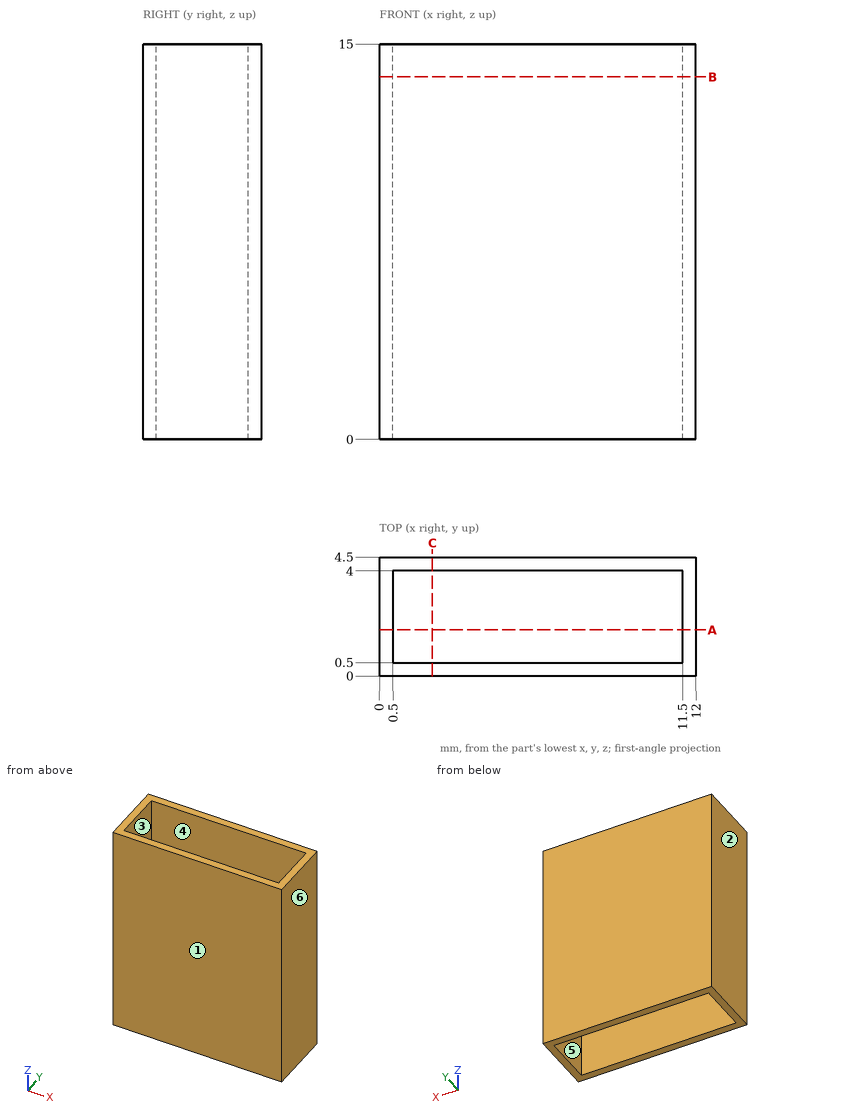
Drawing for the job (mm, zero at the part's lowest x, y, z). A direction names the side the tool comes from. Coordinates: 2 decimals unless noted, no trailing zeros. Write each loop counter-clockwise with the first axis right and the second up, starting at its lowest first coordinate (ties: lowest second). Pieces come first, ordered by that corner, then holes. Notation, with made-up numbers: (84, 62.25) -> (99, 62.25) arc R27 ccw to (99, 91.25) -> close; hole circle Ø9 at (85, -17.75). An arc over 180 degrees is marked (long way). One line per item, written item: value. Start each with the question number.
1) Flat gauge pin, fed straight in: pin 1 Ø3.5 at (x, z) = (8, 6) entering from -Y. Where does the tip first touch, or does it go through?
2) Slice it at C-C on x = 2. Write the cut outline in (y, z), then the cut area to 3 significant figures.
3) Pull direction X, two halves, no side cores. Call the marked faces 1, 2, 3 and 4: +X half, -X half, draft (parallel to the pull), parting line (faces both ways), or undercut.
4) Slice it at A-A on y = 1.75. Write the cut outline in (x, z).
5) Which spindle directions (+Z, -Z, +X, -X, +Y, -Y) get a long thin tool onto all of the face, cutting with end or side? Do the marked faces 5 and 6. Say none if no direction does.
6) Probe probe 1 along X at (y, z) = (0.9, 4); probe 2 along Y at (x, z) = (3.25, 5.75). List the from-to ranges inside material, lowest first.
7) Slice it at B-B on z = 13.75. Write the cut outline in (x, y), then the cut area to 3 significant figures.
Answers follow:
1. pin 1: y = 0
2. outline: (0, 0) -> (0.5, 0) -> (0.5, 15) -> (0, 15) -> close; (4, 0) -> (4.5, 0) -> (4.5, 15) -> (4, 15) -> close
2. area: 15.0 mm2
3. face 1: draft
3. face 2: -X half
3. face 3: undercut
3. face 4: undercut
4. outline: (0, 0) -> (0.5, 0) -> (0.5, 15) -> (0, 15) -> close; (11.5, 0) -> (12, 0) -> (12, 15) -> (11.5, 15) -> close
5. face 5: +Z, -Z
5. face 6: +Z, -Z, +X, +Y, -Y
6. probe 1: 0 to 0.5, 11.5 to 12
6. probe 2: 0 to 0.5, 4 to 4.5
7. outline: (0, 0) -> (12, 0) -> (12, 4.5) -> (0, 4.5) -> close; hole (0.5, 0.5) -> (11.5, 0.5) -> (11.5, 4) -> (0.5, 4) -> close
7. area: 15.5 mm2
